from build123d import *

# Parameters (mm, degrees)
F3_DEPTH = 31.75
F5_DEPTH = 6.444662
F6_R     = 5.08


with BuildPart() as f3:
    # F2 (on Front) → F3 (new body)
    with BuildSketch(Plane.XZ):
        Polygon((444.5, 0), (444.5, 6.443663), (355.548608, 5.631981), (355.6, 0), align=None)
    extrude(amount=F3_DEPTH)

    # F4 (on face) → F5 (cut, through all)
    with BuildSketch(Plane(origin=(0, 0, 0), x_dir=(1, 0, 0), z_dir=(0, 0, -1))):
        with BuildLine():
            Line((434.975, 25.4), (365.073608, 25.4))
            ThreePointArc((365.073608, 25.4), (362.828544, 24.470064), (361.898608, 22.225))
            Line((361.898608, 22.225), (361.898608, 9.525))
            ThreePointArc((361.898608, 9.525), (362.828544, 7.279936), (365.073608, 6.35))
            Line((365.073608, 6.35), (434.975, 6.35))
            ThreePointArc((434.975, 6.35), (437.220064, 7.279936), (438.15, 9.525))
            Line((438.15, 9.525), (438.15, 22.225))
            ThreePointArc((438.15, 22.225), (437.220064, 24.470064), (434.975, 25.4))
        make_face()
    extrude(amount=-F5_DEPTH, mode=Mode.SUBTRACT)

    # F6
    f6_edges = [f3.edges().sort_by_distance(p)[0] for p in [
        (444.5, -31.75, 3.221831),
        (355.574304, -31.75, 2.815991),
        (355.574304, 0, 2.815991),
        (444.5, 0, 3.221831),
    ]]
    fillet(f6_edges, radius=F6_R)


solid = f3.part
The listing builds one solid part. Answer for the finished solid, in the listing's coordinates (mm). A direction names the side the tool comes from. Coordinates: 2 decimals unless noted, no trailing zeros. Order: outer loops, then holes, each group sorted by start corner. A loop starts at its lowest first (then second) coordinate and runs counter-clockwise, first axis right, second up.
Q1. For a pull along X with two mould halves and no side action, classify faces 1 (the face through (357.1, -30.3, 2.8)), 2 (the face through (443.051, -1.528, 3.267)), 3 (the face through (437.24, -24.45, 3.15)), 4 (the face through (399, -26, 0)) as pulls with the +X half, pulls with the -X half, needs draft (parallel to the pull), parting line crosses it, or undercut.
Q2. A cutting plane is placed at C-C, the plane y = -2. Write down the section's boundary in (x, z), and give its area (3 significant figures).
Q3. Which of the six approach directions +Z, -Z, +X, -X, +Y, -Y give full straight-line access (tool end or side, diameter ignored) to faces 5 (the face through (444.5, -16, 3)), 6 (the face through (362.804, -7.305, 2.819))?
Q4. A cutting plane is placed at A-A, the plane y = -11. Write down the section's boundary in (x, z).
Q5. Given P1, Ø1, axis at y = -27.5, z = 1, coming from the -X side; P2, Ø10, axis at x = 421, y = -18.5, coming from the +Z side, each flat-ended and moving along its own axis, determine where each tip first touches the part or whether it passes through.
Q6. Consider line 1 (Y direction, x = 366.5, z = 4.75); line 2 (X direction, y = -17, z = 1.75); line 3 (X direction, y = -7.5, z = 4.75). Determine where each line is inside the solid, lowest interval first.
Q7. A cutting plane is placed at B-B, the plane x = 409. Write down the section's boundary in (y, z).
Answers follow:
1. face 1: pulls with the -X half
1. face 2: pulls with the +X half
1. face 3: undercut
1. face 4: needs draft
2. outline: (356.59, 5.64) - (356.64, 0) - (443.46, 0) - (443.46, 6.43) - close
2. area: 524 mm2
3. face 5: +Z, -Z, +X, +Y, -Y
3. face 6: +Z, -Z
4. outline: (355.55, 5.63) - (355.6, 0) - (361.9, 0) - (361.9, 5.69) - close; (438.15, 0) - (444.5, 0) - (444.5, 6.44) - (438.15, 6.39) - close
5. P1: stops at x = 355.6
5. P2: passes through
6. line 1: y = -31.75 to -25.4, -6.35 to 0
6. line 2: x = 355.58 to 361.9, 438.15 to 444.5
6. line 3: x = 355.56 to 362.63, 437.42 to 444.5
7. outline: (-31.75, 0) - (-25.4, 0) - (-25.4, 6.12) - (-31.75, 6.12) - close; (-6.35, 0) - (0, 0) - (0, 6.12) - (-6.35, 6.12) - close
